The listing builds one solid part. Answer for the finished solid, in the listing's coordinates (mm). Give positions to 0.01 mm unless a question says otherwise; leave off trailing zeros. Loops run counter-clockwise (first coordinate to the right, second up) from the corner with the lowest first, then second, coordinate; pieces in that order, holes last. Notation, with made-up numbers: M -14,76.5 L -4,76.5 A21 cw -4,110.5 Z; hole C 62.25,48 d9. An arc over 180 degrees is marked long. Return JSON: item names as keys, results as strings.
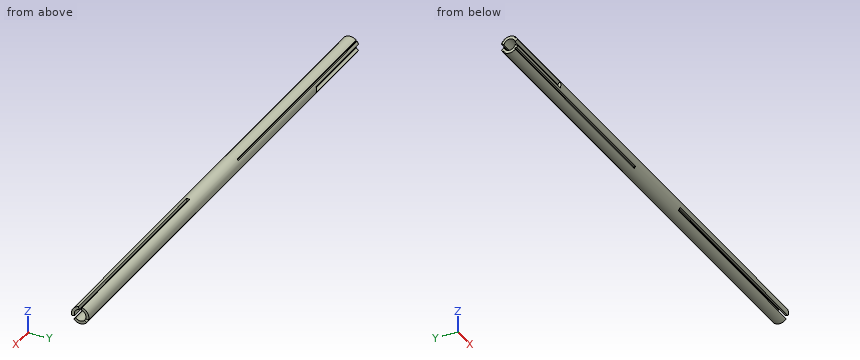
from build123d import *

# Parameters (mm, degrees)
F0_R     = 11
F1_DEPTH = 635
F3_DEPTH = 254
F4_R     = 7.4
F5_DEPTH = 380
F7_DEPTH = 279.4
F8_DEPTH = 100


with BuildPart() as f1:
    # F0 (on Right) → F1 (new body)
    with BuildSketch(Plane.YZ):
        Circle(F0_R)
    extrude(amount=F1_DEPTH)

    # F2 (on face) → F3 (cut)
    with BuildSketch(Plane.YZ.offset(635)):
        with BuildLine():
            ThreePointArc((0, 7.39), (0.724346667, 7.3544151301), (1.4417174797, 7.2480032222))
            Line((1.4417174797, 7.2480032222), (2.1459935422, 10.7886380844))
            ThreePointArc((2.1459935422, 10.7886380844), (0, 11), (-2.1459935422, 10.7886380844))
            Line((-2.1459935422, 10.7886380844), (-1.4417174797, 7.2480032222))
            ThreePointArc((-1.4417174797, 7.2480032222), (-0.724346667, 7.3544151301), (0, 7.39))
        make_face()
        with BuildLine():
            Line((-6.997813657, -2.3754376486), (0, 0))
            Line((0, 0), (-1.4417174797, 7.2480032222))
            ThreePointArc((-1.4417174797, 7.2480032222), (-6.399927734, 3.695), (-6.997813657, -2.3754376486))
        make_face()
        with BuildLine():
            Line((-5.5560961773, -4.8725655736), (0, 0))
            Line((0, 0), (-6.997813657, -2.3754376486))
            ThreePointArc((-6.997813657, -2.3754376486), (-6.399927734, -3.695), (-5.5560961773, -4.8725655736))
        make_face()
        with BuildLine():
            Line((5.5560961773, -4.8725655736), (0, 0))
            Line((0, 0), (-5.5560961773, -4.8725655736))
            ThreePointArc((-5.5560961773, -4.8725655736), (0, -7.39), (5.5560961773, -4.8725655736))
        make_face()
        with BuildLine():
            ThreePointArc((5.5560961773, -4.8725655736), (6.399927734, -3.695), (6.997813657, -2.3754376486))
            Line((6.997813657, -2.3754376486), (0, 0))
            Line((0, 0), (5.5560961773, -4.8725655736))
        make_face()
        with BuildLine():
            ThreePointArc((6.997813657, -2.3754376486), (7.2912942241, -1.2037975484), (7.39, 0))
            ThreePointArc((7.39, 0), (5.7125472504, 4.68816637), (1.4417174797, 7.2480032222))
            Line((1.4417174797, 7.2480032222), (0, 0))
            Line((0, 0), (6.997813657, -2.3754376486))
        make_face()
        with BuildLine():
            Line((0, 0), (1.4417174797, 7.2480032222))
            ThreePointArc((1.4417174797, 7.2480032222), (0.724346667, 7.3544151301), (0, 7.39))
            Line((0, 7.39), (0, 0))
        make_face()
        with BuildLine():
            Line((0, 0), (0, 7.39))
            ThreePointArc((0, 7.39), (-0.724346667, 7.3544151301), (-1.4417174797, 7.2480032222))
            Line((-1.4417174797, 7.2480032222), (0, 0))
        make_face()
        with BuildLine():
            ThreePointArc((-5.5560961773, -4.8725655736), (-6.399927734, -3.695), (-6.997813657, -2.3754376486))
            Line((-6.997813657, -2.3754376486), (-10.4162314244, -3.5358341183))
            ThreePointArc((-10.4162314244, -3.5358341183), (-9.5262794416, -5.5), (-8.2702378823, -7.2528039661))
            Line((-8.2702378823, -7.2528039661), (-5.5560961773, -4.8725655736))
        make_face()
        with BuildLine():
            Line((10.4162314244, -3.5358341183), (6.997813657, -2.3754376486))
            ThreePointArc((6.997813657, -2.3754376486), (6.399927734, -3.695), (5.5560961773, -4.8725655736))
            Line((5.5560961773, -4.8725655736), (8.2702378823, -7.2528039661))
            ThreePointArc((8.2702378823, -7.2528039661), (9.5262794416, -5.5), (10.4162314244, -3.5358341183))
        make_face()
    extrude(amount=-F3_DEPTH, mode=Mode.SUBTRACT)

    # F4 (on face) → F5 (cut)
    with BuildSketch(Plane(origin=(0, 0, 0), x_dir=(0, -1, 0), z_dir=(-1, 0, 0))):
        Circle(F4_R)
    extrude(amount=-F5_DEPTH, mode=Mode.SUBTRACT)

    # F6 (on face) → F7 (cut)
    with BuildSketch(Plane(origin=(0, 0, 0), x_dir=(0, -1, 0), z_dir=(-1, 0, 0))):
        with BuildLine():
            Line((7.1172844619, 8.3871486149), (7.1172844619, 6.972222589))
            Line((7.1172844619, 6.972222589), (8.5081203665, 6.972222589))
            ThreePointArc((8.5081203665, 6.972222589), (7.8446684396, 7.7111073831), (7.1172844619, 8.3871486149))
        make_face()
        with BuildLine():
            ThreePointArc((-9.0388867634, -6.2688536495), (-8.2077799909, -7.3234109281), (-7.2543820773, -8.2688536495))
            Line((-7.2543820773, -8.2688536495), (-7.2051168904, -8.2688536495))
            Line((-7.2051168904, -8.2688536495), (-7.2051168904, -6.2688536495))
            Line((-7.2051168904, -6.2688536495), (-9.0388867634, -6.2688536495))
        make_face()
        with BuildLine():
            ThreePointArc((7.2543820773, -8.2688536495), (8.2077799909, -7.3234109281), (9.0388867634, -6.2688536495))
            Line((9.0388867634, -6.2688536495), (7.1172844619, -6.2688536495))
            Line((7.1172844619, -6.2688536495), (7.1172844619, -8.2688536495))
            Line((7.1172844619, -8.2688536495), (7.2543820773, -8.2688536495))
        make_face()
        with BuildLine():
            Line((-7.2051168904, 6.972222589), (-7.2051168904, 8.3118163235))
            ThreePointArc((-7.2051168904, 8.3118163235), (-7.8851178885, 7.6697402749), (-8.5081203665, 6.972222589))
            Line((-8.5081203665, 6.972222589), (-7.2051168904, 6.972222589))
        make_face()
    extrude(amount=-F7_DEPTH, mode=Mode.SUBTRACT)

    # F6 (on face) → F8 (cut)
    with BuildSketch(Plane(origin=(0, 0, 0), x_dir=(0, -1, 0), z_dir=(-1, 0, 0))):
        with BuildLine():
            ThreePointArc((11, 0), (10.8166538264, 2), (10.2727272727, 3.9333286641))
            ThreePointArc((10.2727272727, 3.9333286641), (8.4387429279, 3.0724521494), (7.2618181818, 1.4233751066))
            ThreePointArc((7.2618181818, 1.4233751066), (7.3653735325, 0.7150333749), (7.4, 0))
            ThreePointArc((7.4, 0), (7.3653735325, -0.7150333749), (7.2618181818, -1.4233751066))
            ThreePointArc((7.2618181818, -1.4233751066), (8.4387429279, -3.0724521494), (10.2727272727, -3.9333286641))
            ThreePointArc((10.2727272727, -3.9333286641), (10.8166538264, -2), (11, 0))
        make_face()
        with BuildLine():
            ThreePointArc((-7.2618181818, -1.4233751066), (-7.4, 0), (-7.2618181818, 1.4233751066))
            ThreePointArc((-7.2618181818, 1.4233751066), (-8.4387429279, 3.0724521494), (-10.2727272727, 3.9333286641))
            ThreePointArc((-10.2727272727, 3.9333286641), (-11, 0), (-10.2727272727, -3.9333286641))
            ThreePointArc((-10.2727272727, -3.9333286641), (-8.4387429279, -3.0724521494), (-7.2618181818, -1.4233751066))
        make_face()
    extrude(amount=-F8_DEPTH, mode=Mode.SUBTRACT)


solid = f1.part
(1) Straight lines are drawn through the part: line 1 along Y through (x, z) = (185, 1); line 2 along Z through (x, y) = (164.5, 0); line 3 along Y through (x, z) = (498.5, 1.25). For each, find the intervals that lie inside material, in ascending order.
Values follow:
{"line 1": "-10.95 to -7.33, 7.33 to 10.95", "line 2": "-11 to -7.4, 7.4 to 11", "line 3": "-10.93 to -7.28, 7.28 to 10.93"}
(2) The part is cut by section C-C (x = 52). Determine the outline of the cut face in (y, z), and give its area (3 significant figures).
Values follow:
{"outline": "M -10.27,-3.93 A11 ccw -9.04,-6.27 L -7.12,-6.27 L -7.12,-8.27 L -7.25,-8.27 A11 ccw 7.25,-8.27 L 7.21,-8.27 L 7.21,-6.27 L 9.04,-6.27 A11 ccw 10.27,-3.93 A4 cw 7.26,-1.42 A7.4 cw -7.26,-1.42 A4 cw Z; M -10.27,3.93 A4 cw -7.26,1.42 A7.4 cw 7.26,1.42 A4 cw 10.27,3.93 A11 ccw 8.51,6.97 L 7.21,6.97 L 7.21,8.31 A11 ccw -7.12,8.39 L -7.12,6.97 L -8.51,6.97 A11 ccw Z", "area": "157 mm²"}
(3) The part is cut by section A-A (x = 188). Determine the outline of the cut face in (y, z), and give its area (3 significant figures).
Values follow:
{"outline": "M -9.04,-6.27 L -7.12,-6.27 L -7.12,-8.27 L -7.25,-8.27 A11 ccw 7.25,-8.27 L 7.21,-8.27 L 7.21,-6.27 L 9.04,-6.27 A11 ccw 8.51,6.97 L 7.21,6.97 L 7.21,8.31 A11 ccw -7.12,8.39 L -7.12,6.97 L -8.51,6.97 A11 ccw Z; hole C 0,0 d14.8", "area": "202 mm²"}
(4) Given pin 1 (1 mm diameter, centred on x = 190.5, y = -8, fed in from -Z); pin 2 (1 mm diameter, centred on x = 331.5, z = 4.5, fed in from +Y); pin 3 (1.5 mm diameter, centred on x = 549.5, z = -3, fed in from +Y), each flat-ended and moving along its own axis, determine where each tip first touches the part or whether it passes through.
Values follow:
{"pin 1": "z = -6.27", "pin 2": "y = 10.25", "pin 3": "y = 10.77"}
(5) The part is cut by section B-B (x = 558). Determine the outline of the cut face in (y, z), and give its area (3 significant figures).
Values follow:
{"outline": "M -10.42,-3.54 L -7,-2.38 A7.39 cw -1.44,7.25 L -2.15,10.79 A11 ccw Z; M -8.27,-7.25 A11 ccw 8.27,-7.25 L 5.56,-4.87 A7.39 cw -5.56,-4.87 Z; M 1.44,7.25 A7.39 cw 7,-2.38 L 10.42,-3.54 A11 ccw 2.15,10.79 Z", "area": "169 mm²"}
